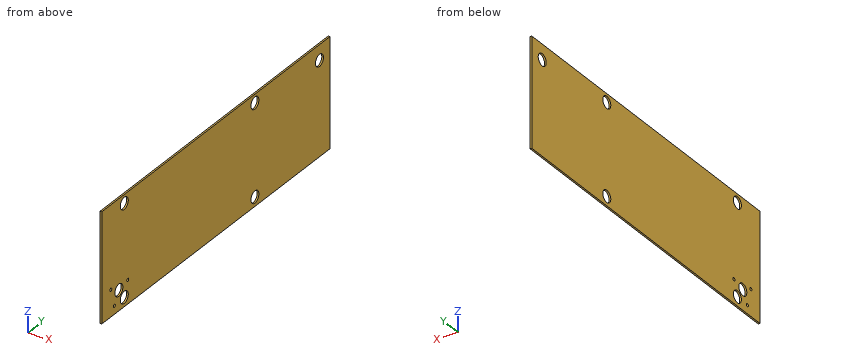
Autodesk Inventor part; units mm, degrees
ref_plane "YZ Plane" through (0, 0, 0) normal (1, 0, 0) x (0, 1, 0)
ref_plane "XZ Plane" through (0, 0, 0) normal (0, 1, 0) x (-1, 0, 0)
ref_plane "XY Plane" through (0, 0, 0) normal (0, 0, 1) x (1, 0, 0)
sketch "Sketch1" plane through (0, 0, 0) normal (1, 0, 0) x (0, 1, 0)
  line L0 (-317.5, 101.6) -> (317.5, 101.6)
  line L1 (317.5, 101.6) -> (317.5, -101.6)
  line L2 (317.5, -101.6) -> (-317.5, -101.6)
  line L3 (-317.5, -101.6) -> (-317.5, 101.6)
  line L4 (-317.5, 101.6) -> (317.5, -101.6) construction
  line L5 (317.5, 101.6) -> (-317.5, -101.6) construction
  point P0 (0, 0)
  dimension "d0" = 635
  dimension "d1" = 203.2
extrude "Plate1" add sketch "Sketch1" along normal blind 3.175
sketch "Sketch2" plane through (3.175, 0, 0) normal (1, 0, 0) x (0, 0, -1)
  circle A0 centre (-85.725, -254.7968) radius 11.1125
  circle A1 centre (84.455, -254.7968) radius 11.1125
  circle A2 centre (-85.725, 108.712) radius 11.1125
  circle A3 centre (84.455, 108.712) radius 11.1125
  circle A4 centre (-85.725, -254.7968) radius 11.938 construction
  circle A5 centre (84.455, -254.7968) radius 11.938 construction
  circle A6 centre (84.455, 108.712) radius 11.938 construction
  circle A7 centre (-85.725, 108.712) radius 11.938 construction
  line L0 (-101.6, -317.5) -> (-101.6, 317.5)
  circle A8 centre (64.0284, -269.8936) radius 12.7 construction
  circle A9 centre (64.0284, -269.8936) radius 11.1125
  point P0 (0, 0)
  point P1 (-138.1252, 190.5)
  dimension "d3" = 22.225
  dimension "d6" = 23.876
  dimension "d7" = 170.18
  dimension "d8" = 15.875
  dimension "d9" = 363.5088
  dimension "d10" = 81.788
  dimension "d11" = 25.4
  dimension "d12" = 25.4
  dimension "d13" = 150.5124
extrude "Cut1" cut sketch "Sketch2" against normal blind 3.175
sketch "Sketch3" plane through (3.175, 0, 0) normal (1, 0, 0) x (0, 0, -1)
  line L0 (-101.6, 269.875) -> (-101.6, 111.125)
  circle A0 centre (-73.025, 288.417) radius 11.1125
  point P0 (0, 0)
  point P1 (-101.6, 190.5)
  dimension "d16" = 22.225
  dimension "d17" = 97.917
  dimension "d18" = 28.575
extrude "Cut2" cut sketch "Sketch3" against normal blind 3.175
sketch "Sketch4" plane through (3.175, 0, 0) normal (1, 0, 0) x (0, 0, -1)
  circle A0 centre (64.0284, -269.8936) radius 11.1125 construction
  line L0 (64.0284, -269.8936) -> (57.8835, -245.2481) construction
  line L1 (64.0284, -269.8936) -> (52.1038, -292.3204) construction
  line L2 (64.0284, -269.8936) -> (86.0254, -282.5936) construction
  line L3 (64.0284, -269.8936) -> (64.0284, -241.3632) construction
  point P0 (0, 0)
  dimension "d21" = 25.4
  dimension "d22" = 14
  dimension "d23" = 28
  dimension "d24" = 60
hole "Hole1" at (3.175, -245.2481, -57.8835) at (3.175, -292.3204, -52.1038) at (3.175, -282.5936, -86.0254) direction (-1, 0, 0) diameter 5.6134 depth 3.175 tip angle 118
equation "\"d14\" = Thickness"
equation "\"d19\" = Thickness"
equation "\"d30\" = Thickness"
equation "\"d2\" = Thickness"
equation "\"BendRadius\" = Thickness"
equation "\"BendReliefWidth\" = Thickness"
equation "\"BendReliefDepth\" = 0.5 * Thickness"
equation "\"CornerReliefSize\" = 4 * Thickness"
equation "\"MinimumRemnant\" = 2 * Thickness"
equation "\"TransitionRadius\" = BendRadius"
equation "\"JacobiRadiusSize\" = BendRadius"
equation "\"GapSize\" = Thickness"
properties part number "PLATE,BACK" material "Aluminum 6061"
Input: part model. Units: mm. Frame: model coordinates. Give positions to 0.01 mm unless a question says otherwise; leave off trailing zeros. Order: outer loops, then holes, each group sorted by start corner. A loop starts at its lowest first (then second) coordinate and runs counter-clockwise, first axis right, second up.
Q1. Contact query for flat-ended pins moving along their axis: pin 1 Ø1.5 at (y, z) = (195, 54) entering from -X; pin 2 Ø18 at (y, z) = (-254.8, -84.46) entering from +X. Output: stop coordinate, or through.
Checked values:
pin 1: stops at x = 0
pin 2: passes through
Q2. Ray query, probe 1 along Z at (x, y) = (1.75, -253); probe 2 along Z at (x, y) = (2.95, -251); probe 3 along Y at (x, z) = (2.65, 83). Return the intervals inside material, ascending.
Checked values:
probe 1: z = -101.6 to -95.42, -73.49 to 74.76, 96.69 to 101.6
probe 2: z = -101.6 to -94.9, -74.01 to 75.28, 96.17 to 101.6
probe 3: y = -317.5 to -265.57, -244.02 to 97.94, 119.49 to 283.52, 293.31 to 317.5
Q3. Section A-A on z = -67.5. Output: boundary loops of the cut face in (x, y) (3 decimals), and give its area (3 significant figures).
Checked values:
outline: (0, -317.5) - (3.175, -317.5) - (3.175, -280.45) - (0, -280.45) - close; (0, -259.337) - (3.175, -259.337) - (3.175, 317.5) - (0, 317.5) - close
area: 1,950 mm2
Q4. Section B-B on x = 2.4. State how many separate pieces and enclosed holes the cut face has, and give its area (3 significant figures).
Checked values:
separate pieces: 1
enclosed holes: 9
area: 127,000 mm2
